For this review, take the finished solid that the model builds, in its own axes (mm). A direction names the side the tool comes from. Round coordinates to 2 decimals unless told otherwise and drop trailing zeros. Loops run counter-clockwise (first coordinate to the right, second up) from the corner with the lowest first, then second, coordinate; pieces in that order, holes last.
1. Tool access review of faces 3 (the flat face through (140, 0, -46)), 4 (the cylindrical face through (-10, 0, -70)), 5 (the cylindrical face through (4.425, -39.923, -20.765)): name each direction out of +Z, -Z, +X, -X, +Y, -Y from which nothing blocks a thin tool from reaching the whole face with its end or side.
2. Consider section A-A on y = 0. State the section outline as (x, z) points, then the cut area to 3 significant figures.
3. Consider section C-C on x = -24.5. State the section outline as (y, z) points.
4. Consider section D-D on z = -70. State the section outline as (x, y) points, then the cut area to 3 significant figures.
5. Draft analysis for pull direction Z (two halves, no side actions). For faces 1 (the flat face through (-135, 1, 1)), 2 (the cylindrical face through (-117.83, -9.76, -52.05)), state which applies: released by +Z, released by -Z, zero draft, split by the parting line, or undercut.
6. Consider section B-B on x = 13. State the section outline as (y, z) points, then the cut area to 3 significant figures.
7. Clearance check with flat-ended pins moving along their axes: pin 1 Ø5 at (y, z) = (5, -6.5) entering from +X; pin 2 Ø12 at (x, y) = (-7.5, 3.5) entering from +Z; pin 3 Ø8 at (x, z) = (31.5, 33.5) entering from -Y. State where each tip first meets the part, or that it passes through.
8. To check wall thickness, follow line 1 along Y through (x, z) = (-120, -56); line 2 along Z through (x, y) = (-75, 38); line 3 along X through (y, z) = (0, -54). State the ranges of each line that lie inside material, in increasing order.
from build123d import *

# Parameters (mm, degrees)
EXTRUDE_1_DEPTH     = 140
FILLET_1_R          = 3
SKETCH_3_R          = 45
CUT_EXTRUDE_1_DEPTH = 275
SKETCH_4_R          = 10
CUT_EXTRUDE_2_DEPTH = 30


with BuildPart() as part:
    # Эскиз1 → Бобышка-Вытянуть1 (new, symmetric)
    with BuildSketch(Plane(origin=(0, 0, 0), x_dir=(0, 0, -1), z_dir=(1, 0, 0))):
        with BuildLine():
            Line((60, -50), (60, 50))
            Line((60, 50), (48, 50))
            ThreePointArc((48, 50), (45.878679656, 49.121320344), (45, 47))
            Line((45, 47), (45, 44.665422868))
            ThreePointArc((45, 44.665422868), (40.403851774, 37.42568578), (31.896551724, 38.504674886))
            ThreePointArc((31.896551724, 38.504674886), (-50, 0), (31.896551724, -38.504674886))
            ThreePointArc((31.896551724, -38.504674886), (40.403851774, -37.42568578), (45, -44.665422868))
            Line((45, -44.665422868), (45, -47))
            ThreePointArc((45, -47), (45.878679656, -49.121320344), (48, -50))
            Line((48, -50), (60, -50))
        make_face()
    extrude(amount=EXTRUDE_1_DEPTH, both=True)

    # Скругление1
    fillet_1_edges = [part.edges().sort_by_distance(p)[0] for p in [
        (-140, 0, 50),
        (-140, 37.42568578, -40.403851774),
        (-140, 45.832711434, -45),
        (-140, 49.121320344, -45.878679656),
        (-140, 50, -54),
        (-140, -50, -54),
        (-140, -49.121320344, -45.878679656),
        (140, 50, -54),
        (140, 49.121320344, -45.878679656),
        (140, 45.832711434, -45),
        (140, 37.42568578, -40.403851774),
        (140, 0, 50),
        (140, -37.42568578, -40.403851774),
        (140, -45.832711434, -45),
        (140, -49.121320344, -45.878679656),
        (140, -50, -54),
        (-140, -45.832711434, -45),
        (-140, -37.42568578, -40.403851774),
    ]]
    fillet(fillet_1_edges, radius=FILLET_1_R)

    # Эскиз2 → Повернуть1 (revolve)
    with BuildSketch(Plane(origin=(0, 0, 0), x_dir=(0, 0, -1), z_dir=(1, 0, 0)), mode=Mode.PRIVATE) as revolve_1_sk:
        with BuildLine():
            Line((60, 0), (60, 10))
            Line((60, 10), (80, 10))
            Line((80, 10), (80, 20))
            ThreePointArc((80, 20), (87.360679775, 11.180339887), (90, 0))
            Line((90, 0), (60, 0))
        make_face()
    revolve(revolve_1_sk.sketch.rotate(Axis((0, 0, 60.403427692), (0, 0, -1)), 90), axis=Axis((0, 0, 60.403427692), (0, 0, -1)))

    # Эскиз3 → Вырез-Вытянуть1 (cut)
    with BuildSketch(Plane(origin=(140, 0, 0), x_dir=(0, 0, -1), z_dir=(1, 0, 0))):
        Circle(SKETCH_3_R)
    extrude(amount=-CUT_EXTRUDE_1_DEPTH, mode=Mode.SUBTRACT)

    # Эскиз4 → Вырез-Вытянуть2 (cut)
    with BuildSketch(Plane(origin=(0, 0, -60), x_dir=(-1, 0, 0), z_dir=(0, 0, -1))):
        with Locations((120, 0)):
            Circle(SKETCH_4_R)
    extrude(amount=-CUT_EXTRUDE_2_DEPTH, mode=Mode.SUBTRACT)


solid = part.part
Resolved:
1. face 3: +Z, -Z, +X, +Y, -Y
1. face 4: none
1. face 5: +X
2. outline: (-140, -60) - (-130, -60) - (-130, -45) - (-135, -45) - (-135, 45) - (140, 45) - (140, 47) arc R3 ccw to (137, 50) - (-137, 50) arc R3 ccw to (-140, 47) - close; (-110, -60) - (-10, -60) - (-10, -80) - (-20, -80) arc R25 ccw to (20, -80) - (10, -80) - (10, -60) - (140, -60) - (140, -45) - (-110, -45) - close
2. area: 6,430 mm2
3. outline: (-50, -60) - (50, -60) - (50, -48) arc R3 ccw to (47, -45) - (44.67, -45) arc R8 cw to (38.5, -31.9) arc R50 ccw (long way) to (-38.5, -31.9) arc R8 cw to (-44.67, -45) - (-47, -45) arc R3 ccw to (-50, -48) - close; hole circle Ø90 at (0, 0)
4. outline: circle Ø20 at (0, 0)
4. area: 314 mm2
5. face 1: undercut
5. face 2: zero draft
6. outline: (-50, -60) - (50, -60) - (50, -48) arc R3 ccw to (47, -45) - (44.67, -45) arc R8 cw to (38.5, -31.9) arc R50 ccw (long way) to (-38.5, -31.9) arc R8 cw to (-44.67, -45) - (-47, -45) arc R3 ccw to (-50, -48) - close; (-15.2, -80) arc R21.35 ccw to (15.2, -80) - close; hole circle Ø90 at (0, 0)
6. area: 3,150 mm2
7. pin 1: stops at x = -135
7. pin 2: stops at z = 50
7. pin 3: stops at y = -40.37
8. line 1: y = -50 to -10, 10 to 50
8. line 2: z = -60 to -41.42, -32.58 to -24.1, 24.1 to 32.5
8. line 3: x = -140 to -130, -110 to 140
